Here's how the part is built. I have some questions about the finished solid (model axes, mm). A direction names the side the tool comes from. Round coordinates to 2 decimals unless told otherwise and drop trailing zeros. Write each loop counter-clockwise with the first axis right and the second up, starting at its lowest first coordinate (ties: lowest second). Pieces come first, ordered by that corner, then holes. Notation, with made-up numbers: (50.5, -13.75) - (62.5, -13.75) arc R19 cw to (62.5, 12.25) - close; hole circle Ø6 at (1, 61). An arc over 180 degrees is marked (long way). Use one line per item in the form item = value. Start each with the question number.
1. Will these pins go through, and if not, where does the flat tip stop? pin 1 (1 mm diameter, centred on x = 10, y = 1.5, fed in from +Z); pin 2 (1.5 mm diameter, centred on x = 9, y = -3, fed in from +Z); pin 3 (1 mm diameter, centred on x = -11, z = 9.5, fed in from +Y).
2. If I drill on line 1 along Y through (x, z) = (-0.5, 7.75); line 2 along X through (y, z) = (-3, 3.5); line 3 along Z through (x, y) = (-1, 1), over which ranges is the centre line in solid material (lowest first)?
3. Which directions (+Z, -Z, +X, -X, +Y, -Y) give clear straight access to the entire face, cutting with the end or side of a thin tool? Please do faces 1 (the cylindrical face through (24.1, -7.64, 5.54)), 2 (the flat face through (0, 3.247, 6)).
4. I want a section at C-C, the plane x = 18.75. List the corners of the cut face in (y, z) for me, plus the area to 3 significant figures.
5. We'd pull the mould along Y, two halves only. Please class faces 3 (the flat face through (0, 0, 3)), 4 (the flat face through (0, 0, 0)), 5 (the flat face through (0, -8.5, 5)): +Y half, -Y half, draft (parallel to the pull), parting line (faces both ways), or undercut.
6. I want a section at A-A, the plane z = 5.75. List the corners of the cut face in (x, y) for me, plus the area to 3 significant figures.
7. I want a section at D-D, the plane z = 10.25. List the corners of the cut face in (x, y) for me, plus the area to 3 significant figures.
8. I want a section at B-B, the plane y = 0. List the corners of the cut face in (x, z) for me, plus the area to 3 significant figures.
```python
from build123d import *

# Parameters (mm, degrees)
F0_W     = 50
F0_H     = 17
F1_DEPTH = 8
F2_R     = 2.75
F3_DEPTH = 6
F2_W     = 23
F2_H     = 6.494846
F4_DEPTH = 5
F5_R     = 3
F6_SIZE  = 1


with BuildPart() as f1:
    # F0 (on Top) → F1 (new body)
    with BuildSketch(Plane.XY):
        Rectangle(F0_W, F0_H)
    extrude(amount=F1_DEPTH)

    # F2 (on face) → F3 (join)
    with BuildSketch(Plane.XY.offset(8)):
        with Locations((-18.75, 0)):
            Circle(F2_R)
        with Locations((18.75, 0)):
            Circle(F2_R)
    extrude(amount=F3_DEPTH)

    # F2 (on face) → F4 (cut)
    with BuildSketch(Plane.XY.offset(8)):
        Rectangle(F2_W, F2_H)
    extrude(amount=-F4_DEPTH, mode=Mode.SUBTRACT)

    # F5
    f5_edges = [f1.edges().sort_by_distance(p)[0] for p in [
        (-25, -8.5, 4),
        (25, -8.5, 4),
        (-25, 8.5, 4),
        (25, 8.5, 4),
        (0, 8.5, 0),
        (25, 0, 0),
        (0, -8.5, 0),
        (-25, 0, 0),
    ]]
    fillet(f5_edges, radius=F5_R)

    # F6
    f6_edges = [f1.edges().sort_by_distance(p)[0] for p in [
        (-21.5, 0, 14),
        (16, 0, 14),
    ]]
    chamfer(f6_edges, length=F6_SIZE)


solid = f1.part
```
Model answer:
q1.pin_1 = 3
q1.pin_2 = 8
q1.pin_3 = through
q2.line_1 = -8.5 to -3.25, 3.25 to 8.5
q2.line_2 = -25 to -11.5, 11.5 to 25
q2.line_3 = 0 to 3
q3.face_1 = +Z, -Z, +X, -Y
q3.face_2 = +Z
q4.outline = (-8.5, 3) arc R3 ccw to (-5.5, 0) - (5.5, 0) arc R3 ccw to (8.5, 3) - (8.5, 8) - (2.75, 8) - (2.75, 13) - (1.75, 14) - (-1.75, 14) - (-2.75, 13) - (-2.75, 8) - (-8.5, 8) - close
q4.area = 164 mm2
q5.face_3 = undercut
q5.face_4 = draft
q5.face_5 = -Y half
q6.outline = (-25, -5.5) arc R3 ccw to (-22, -8.5) - (22, -8.5) arc R3 ccw to (25, -5.5) - (25, 5.5) arc R3 ccw to (22, 8.5) - (-22, 8.5) arc R3 ccw to (-25, 5.5) - close; hole (-11.5, -3.25) - (11.5, -3.25) - (11.5, 3.25) - (-11.5, 3.25) - close
q6.area = 693 mm2
q7.outline = circle Ø5.5 at (-18.75, 0); circle Ø5.5 at (18.75, 0)
q7.area = 47.5 mm2
q8.outline = (-25, 3) arc R3 ccw to (-22, 0) - (22, 0) arc R3 ccw to (25, 3) - (25, 8) - (21.5, 8) - (21.5, 13) - (20.5, 14) - (17, 14) - (16, 13) - (16, 8) - (11.5, 8) - (11.5, 3) - (-11.5, 3) - (-11.5, 8) - (-16, 8) - (-16, 13) - (-17, 14) - (-20.5, 14) - (-21.5, 13) - (-21.5, 8) - (-25, 8) - close
q8.area = 345 mm2
